Verification items for the finished model (mm, model axes). A direction names the side the tool comes from. Give positions to 0.01 mm unless a question says otherwise; leave off trailing zeros. Write each loop counter-clockwise with the first axis right and the second up, starting at its lowest first coordinate (ties: lowest second). Pieces come first, ordered by that corner, then holes. Notation, with made-up numbers: M -37,-32 L -12,-32 A17 cw -12,-8 Z; hole C -3.75,40 d2. An arc over 180 degrees is marked long. Answer as a JSON object with one key per item and string values.
```python
from build123d import *

# Parameters (mm, degrees)
SKETCH2_W           = 100
SKETCH2_H           = 3
BOSS_EXTRUDE2_DEPTH = 150
SKETCH3_W           = 12.3
SKETCH3_H           = 32.2
BOSS_EXTRUDE3_DEPTH = 22.5
SKETCH4_R           = 5.5
BOSS_EXTRUDE4_DEPTH = 3
SKETCH10_R          = 2.5
BOSS_EXTRUDE5_DEPTH = 3.2


with BuildPart() as part:
    # Sketch2 → Boss-Extrude2 (new body)
    with BuildSketch(Plane.XY):
        Rectangle(SKETCH2_W, SKETCH2_H)
    extrude(amount=-BOSS_EXTRUDE2_DEPTH)

    # Sketch3 → Boss-Extrude3 (add)
    with BuildSketch(Plane(origin=(0, 0, 0), x_dir=(1, 0, 0), z_dir=(0, 1, 0))):
        with Locations((0, 75)):
            Rectangle(SKETCH3_W, SKETCH3_H)
    extrude(amount=BOSS_EXTRUDE3_DEPTH)

    # Sketch4 → Boss-Extrude4 (add)
    with BuildSketch(Plane(origin=(0, 22.5, 0), x_dir=(1, 0, 0), z_dir=(0, 1, 0))):
        with Locations((0, 64.4)):
            Circle(SKETCH4_R)
    extrude(amount=BOSS_EXTRUDE4_DEPTH)

    # Sketch10 → Boss-Extrude5 (add)
    with BuildSketch(Plane(origin=(0, 25.5, 0), x_dir=(1, 0, 0), z_dir=(0, 1, 0))):
        with Locations((0, 64.4)):
            Circle(SKETCH10_R)
    extrude(amount=BOSS_EXTRUDE5_DEPTH)


solid = part.part
```
1) Section check A-A on z = -72.5. Record the boundary of the cut face in (x, y), and give its area (3 significant figures).
Completed:
{"outline": "M -50,-1.5 L 50,-1.5 L 50,1.5 L 6.15,1.5 L 6.15,22.5 L -6.15,22.5 L -6.15,1.5 L -50,1.5 Z", "area": "558 mm2"}
2) Thickness scan on L1, parallel to Y at x = 27, z = -5.5; L2, parallel to X at y = 2, z = -61; L3, parallel to Z at x = 5.5, y = 22. Record the ranges inside material, lowest first.
Completed:
{"L1": "y = -1.5 to 1.5", "L2": "x = -6.15 to 6.15", "L3": "z = -91.1 to -58.9"}
3) Access from +Z, -Z, +X, -X, +Y, -Y to the whole of each face (thin tool, end or side, straight path). Record for faces 1 (the face through (-3, 25.5, -64)), 2 (the face through (6.15, 12, -75)), 3 (the face through (0, 12, -58.9)).
Completed:
{"face 1": "+Y", "face 2": "+Z, -Z, +X, +Y", "face 3": "+Z, +X, -X, +Y"}
4) Section check B-B on y = 4.5. Record the boundary of the cut face in (x, z), and give its area (3 significant figures).
Completed:
{"outline": "M -6.15,-91.1 L 6.15,-91.1 L 6.15,-58.9 L -6.15,-58.9 Z", "area": "396 mm2"}
5) Go/stop test with flat-tipped pins: pin 1 (17 mm diameter, centred on y = 14.5, z = -81.5, fed in from +X); pin 2 (10 mm diameter, centred on x = -2.5, z = -74, fed in from +Y); pin 3 (3.5 mm diameter, centred on x = 0, y = 11, fed in from -Z). Record where each tip stops, or that it passes through.
Completed:
{"pin 1": "stops at x = 6.15", "pin 2": "stops at y = 25.5", "pin 3": "stops at z = -91.1"}
6) Section check C-C on x = -18.5. Record the boundary of the cut face in (y, z), and give its area (3 significant figures).
Completed:
{"outline": "M -1.5,-150 L 1.5,-150 L 1.5,0 L -1.5,0 Z", "area": "450 mm2"}
